Could you check a few things on this drawing? It's one solid part, dimensions in mm from its lowest x, y, z. Give positions to 0.01 mm unless a question says otherwise; leave off trailing zeros. Order: outer loops, then holes, each group sorted by start corner. A loop starts at its lowest first (then second) coordinate and runs counter-clockwise, first axis right, second up. Notation, with made-up numbers: (-5, 72.5) -> (41, 72.5) arc R22 cw to (41, 89.5) -> close; hole circle Ø3 at (34.5, 67). An arc over 180 degrees is marked (long way). Answer as a JSON object with one key per item and string values.
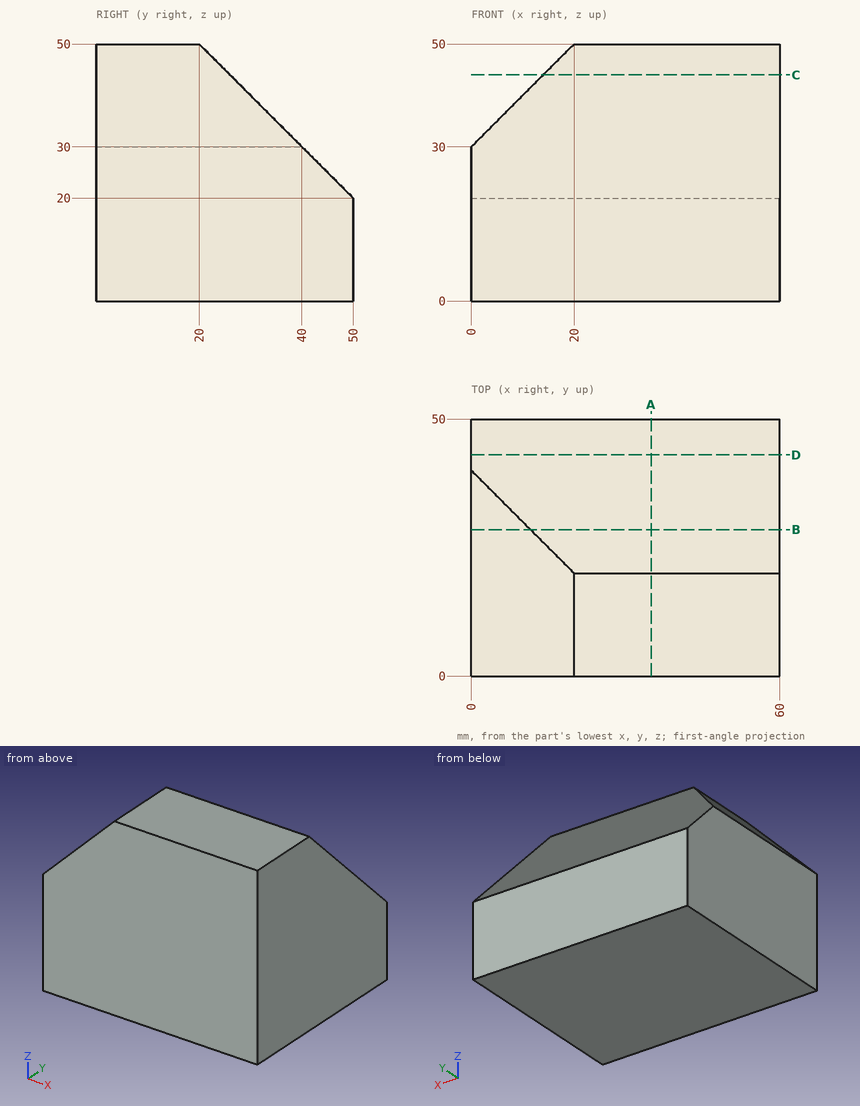
1. If we section it at A-A on x = 35: Please give me the cut outline in (y, z), then the cut area to 3 significant figures.
Worked answers:
{"outline": "(0, 0) -> (50, 0) -> (50, 20) -> (20, 50) -> (0, 50) -> close", "area": "2,050 mm²"}
2. If we section it at C-C on z = 44: Please give me the cut outline in (x, y).
Worked answers:
{"outline": "(14, 0) -> (60, 0) -> (60, 26) -> (14, 26) -> close"}
3. Will this pin go through, and if not, where does the flat tip stop? pin 1 Ø4 at (x, z) = (24, 24.5) entering from +Y.
Worked answers:
{"pin 1": "y = 47.5"}
4. If we section it at B-B on y = 28.5: Please give me the cut outline in (x, z), then the cut area to 3 significant figures.
Worked answers:
{"outline": "(0, 0) -> (60, 0) -> (60, 41.5) -> (11.5, 41.5) -> (0, 30) -> close", "area": "2,420 mm²"}
5. Please list where these lines run through material, in increasing order: L1, parallel to Y at x = 11.5, z = 40; L2, parallel to Z at x = 7.5, y = 10.5; L3, parallel to Z at x = 15, y = 34.
Worked answers:
{"L1": "0 to 30", "L2": "0 to 37.5", "L3": "0 to 36"}
6. If we section it at D-D on y = 43: Please give me the cut outline in (x, z), then the cut area to 3 significant figures.
Worked answers:
{"outline": "(0, 0) -> (60, 0) -> (60, 27) -> (0, 27) -> close", "area": "1,620 mm²"}
